Check sheet for the modelled part. Datum: model origin and axes. Units: mm. Round coordinates to 2 decimals unless told otherwise and drop trailing zeros. Write each loop counter-clockwise with the first axis right and the second up, starting at its lowest first coordinate (ties: lowest second). Pieces come first, ordered by that corner, then holes.
Item 1: Section check B-B, the plane y = -24. Record the cut outline in (x, z), plus the area to 3 significant figures.
Item 2: Depth check by flat-ended pin: pin 1 (4 mm diameter, centred on x = -91, z = 43.5, fed in from +Y); pin 2 (6 mm diameter, centred on x = -20, y = -10, fed in from +Z). Enter the tip coordinate at first touch or a pass-through.
Item 3: Release check for a two-part mould opening along X. For faces 1 (the flat face through (-63, -30, 143)), 2 (the cylindrical face through (-25, -10, 147)), 3 (the flat face through (-105, -15, 143)) record: pulls with the +X half, pulls with the -X half, needs draft (parallel to the pull), parting line crosses it, or undercut.
Item 4: Section check A-A, the plane z = 236.5. Record the cut outline in (x, y).
Item 5: Material ranges on line 1 along Y through (x, z) = (-20, 195); line 2 along X through (y, z) = (-14.5, 223); line 3 along X through (y, z) = (-18.5, 84.5), recorded low to high.
from build123d import *

# Parameters (mm, degrees)
EXTRUDE_1_DEPTH     = 290
SKETCH_2_R          = 5
CUT_EXTRUDE_1_DEPTH = 291


with BuildPart() as part:
    # 草图1 → 凸台-拉伸1 (new body)
    with BuildSketch(Plane.XY):
        with BuildLine():
            Line((0, 0), (-105, 0))
            Line((-105, 0), (-105, -30))
            Line((-105, -30), (-20, -30))
            ThreePointArc((-20, -30), (-5.857864376, -24.142135624), (0, -10))
            Line((0, -10), (0, 0))
        make_face()
    extrude(amount=EXTRUDE_1_DEPTH)

    # 草图2 → 切除-拉伸1 (cut, through all)
    with BuildSketch(Plane.XY.offset(290)):
        with Locations((-20, -10)):
            Circle(SKETCH_2_R)
    extrude(amount=-CUT_EXTRUDE_1_DEPTH, mode=Mode.SUBTRACT)


solid = part.part
Values found:
1. outline: (-105, 0) - (-5.72, 0) - (-5.72, 290) - (-105, 290) - close
1. area: 28,800 mm2
2. pin 1: stops at y = 0
2. pin 2: passes through
3. face 1: needs draft
3. face 2: undercut
3. face 3: pulls with the -X half
4. outline: (-105, -30) - (-20, -30) arc R20 ccw to (0, -10) - (0, 0) - (-105, 0) - close; hole circle Ø10 at (-20, -10)
5. line 1: y = -30 to -15, -5 to 0
5. line 2: x = -105 to -22.18, -17.82 to -0.51
5. line 3: x = -105 to -1.9
